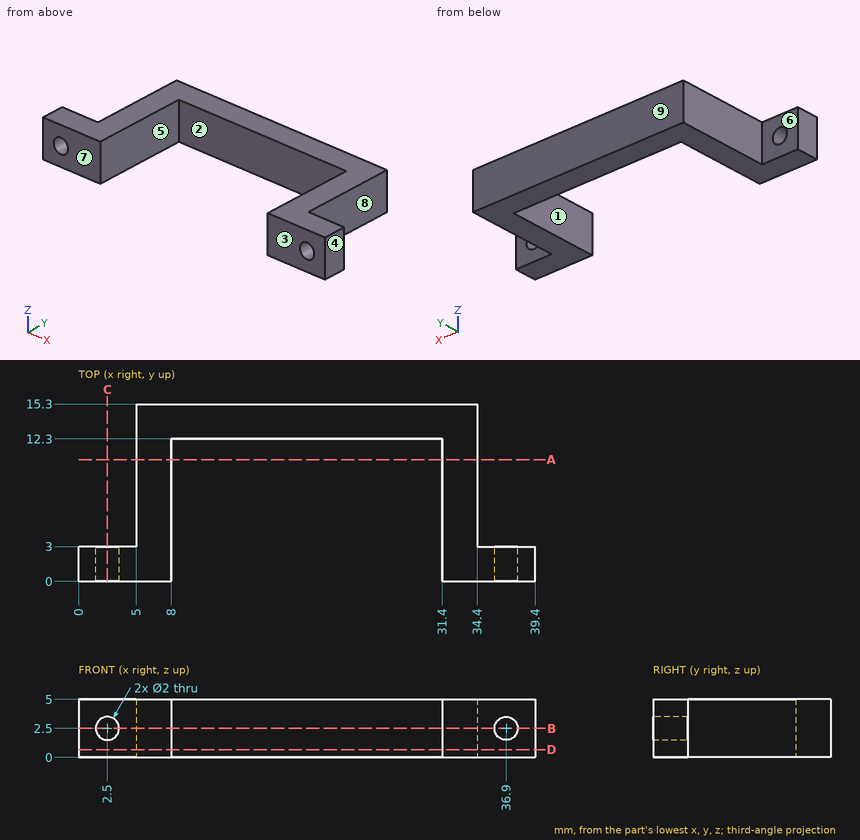
Answer from the drawing. Dimensions are ordinates in mm from the lowest x, y and z of the part. A direction names the side the tool comes from. Give positions to 0.01 mm unless a question says otherwise; leave off trailing zeros. Order: outer loops, then holes, each group sorted by start corner. A loop starts at its lowest first (then second) coordinate and runs counter-clockwise, first axis right, second up.
(1) For a pull along X with two mould halves and no side action, classify the marked faces 1, 2, 3 and 4 as released by +X, released by -X, zero draft, split by the parting line, or undercut.
(2) Find section D-D (z = 0.65). Give the vertices of the cut face in (x, y), plus the area to 3 significant figures.
(3) Given pin 1 (1.5 mm diameter, centred on y = 10, z = 3.5, fed in from -X); pin 2 (1 mm diameter, centred on x = 21, z = 2, fed in from -Y); pin 3 (1.6 mm diameter, centred on x = 2.5, z = 2.5, fed in from -Y); pin 4 (1.5 mm diameter, centred on x = 36.5, z = 2.5, fed in from +Y), each flat-ended and moving along its own axis, determine where each tip first touches the part or whether it passes through.
(4) Find section A-A (y = 10.5). Give the vertices of the cut face in (x, z).
(5) Find section B-B (z = 2.5). Give the vertices of the cut face in (x, y), plus the area to 3 significant figures.
(6) Find section C-C (x = 2.5). Give the vertices of the cut face in (y, z).
(7) For the marked faces 5, 6, 7, 8 and 9, determine the directions among +Z, -Z, +X, -X, +Y, -Y from which every point of the face is accessible in a straight line to the end or side of a thin tool.
(8) Straight lines are drawn through the part: L1, parallel to X at y = 1.45, z = 2.5; L2, parallel to Z at x = 2.5, y = 2.05; L3, parallel to X at y = 8, z = 3.5. For each, find the intervals that lie inside material, in ascending order.
Result sheet:
1. face 1: undercut
1. face 2: undercut
1. face 3: zero draft
1. face 4: released by +X
2. outline: (0, 0) - (8, 0) - (8, 12.3) - (31.4, 12.3) - (31.4, 0) - (39.4, 0) - (39.4, 3) - (34.4, 3) - (34.4, 15.3) - (5, 15.3) - (5, 3) - (0, 3) - close
2. area: 192 mm2
3. pin 1: stops at x = 5
3. pin 2: stops at y = 12.3
3. pin 3: passes through
3. pin 4: stops at y = 3
4. outline: (5, 0) - (8, 0) - (8, 5) - (5, 5) - close; (31.4, 0) - (34.4, 0) - (34.4, 5) - (31.4, 5) - close
5. outline: (0, 0) - (1.5, 0) - (1.5, 3) - (0, 3) - close; (3.5, 0) - (8, 0) - (8, 12.3) - (31.4, 12.3) - (31.4, 0) - (35.9, 0) - (35.9, 3) - (34.4, 3) - (34.4, 15.3) - (5, 15.3) - (5, 3) - (3.5, 3) - close; (37.9, 0) - (39.4, 0) - (39.4, 3) - (37.9, 3) - close
5. area: 180 mm2
6. outline: (0, 0) - (3, 0) - (3, 1.5) - (0, 1.5) - close; (0, 3.5) - (3, 3.5) - (3, 5) - (0, 5) - close
7. face 5: +Z, -Z, -Y
7. face 6: +Z, -Z, -X, +Y
7. face 7: +Z, -Z, +X, -X, -Y
7. face 8: +Z, -Z, +X, +Y
7. face 9: +Z, -Z, +X, -X, +Y
8. L1: x = 0 to 1.5, 3.5 to 8, 31.4 to 35.9, 37.9 to 39.4
8. L2: z = 0 to 1.5, 3.5 to 5
8. L3: x = 5 to 8, 31.4 to 34.4
